from build123d import *

# Parameters (mm, degrees)
F0_R     = 6.5
F1_DEPTH = 60
F3_ANGLE = 90


# Not quite as in the source:
# - a feature names something its author has since deleted; it is built from what else it names


with BuildPart() as f1:
    # F0 (on Front) → F1 (new body)
    with BuildSketch(Plane.XZ):
        with BuildLine():
            Line((-11.7955299893, 45.4649311314), (-27.0527510662, 12.5336819647))
            ThreePointArc((-27.0527510662, 12.5336819647), (-29.8151727119, 0), (-27.0527510662, -12.5336819647))
            Line((-27.0527510662, -12.5336819647), (-11.7955299893, -45.4649311314))
            ThreePointArc((-11.7955299893, -45.4649311314), (0, -53), (11.7955299893, -45.4649311314))
            Line((11.7955299893, -45.4649311314), (27.0527510662, -12.5336819647))
            ThreePointArc((27.0527510662, -12.5336819647), (29.8151727119, 0), (27.0527510662, 12.5336819647))
            Line((27.0527510662, 12.5336819647), (11.7955299893, 45.4649311314))
            ThreePointArc((11.7955299893, 45.4649311314), (0, 53), (-11.7955299893, 45.4649311314))
        make_face()
        with Locations((0, -40)):
            Circle(F0_R, mode=Mode.SUBTRACT)
        with BuildLine():
            ThreePointArc((17.9448621018, -5.4354782815), (-18.75, 0), (17.9448621018, 5.4354782815))
            ThreePointArc((17.9448621018, 5.4354782815), (24.1748678936, 5.401139318), (27.28, 0))
            ThreePointArc((27.28, 0), (24.1748678936, -5.401139318), (17.9448621018, -5.4354782815))
        make_face(mode=Mode.SUBTRACT)
        with Locations((0, 40)):
            Circle(F0_R, mode=Mode.SUBTRACT)
        with BuildLine():
            ThreePointArc((17.9448621018, 5.4354782815), (18.5476233573, 2.7473929089), (18.75, 0))
            ThreePointArc((18.75, 0), (18.5476233573, -2.7473929089), (17.9448621018, -5.4354782815))
            ThreePointArc((17.9448621018, -5.4354782815), (24.1748678936, -5.401139318), (27.28, 0))
            ThreePointArc((27.28, 0), (24.1748678936, 5.401139318), (17.9448621018, 5.4354782815))
        make_face()
    extrude(amount=F1_DEPTH)


with BuildPart() as f2:
    # F0 (on Front) → F2 (revolve)
    with BuildSketch(Plane.XZ):
        with BuildLine():
            ThreePointArc((78.6849431597, 21.03), (68.9626292834, 15.8333148696), (70.0431715295, 26.8042470045))
            Line((70.0431715295, 26.8042470045), (65.4349431597, 24.8954563152))
            Line((65.4349431597, 24.8954563152), (65.4349431597, 0))
            Line((65.4349431597, 0), (79.4349431597, 0))
            Line((79.4349431597, 0), (79.4349431597, 24.8954563152))
            Line((79.4349431597, 24.8954563152), (74.8267146878, 26.8042470468))
            ThreePointArc((74.8267146878, 26.8042470468), (77.6316282594, 24.5023139222), (78.6849431597, 21.03))
        make_face()
        with BuildLine():
            ThreePointArc((74.8267146878, 26.8042470468), (72.4349431044, 27.28), (70.0431715295, 26.8042470045))
            ThreePointArc((70.0431715295, 26.8042470045), (68.9626292834, 15.8333148696), (78.6849431597, 21.03))
            ThreePointArc((78.6849431597, 21.03), (77.6316282594, 24.5023139222), (74.8267146878, 26.8042470468))
        make_face()
    revolve(axis=Axis((72.4349431597, 0, 0), (1, 0, 0)))


with BuildPart() as f2_1:
    # F3: moved
    add(f2.part.rotate(Axis((72.4349431597, 0, 17.3734594136), (0, 0, 1)), F3_ANGLE))


with BuildPart() as f2_2:
    # F4: moved
    add(f2_1.part.moved(Location((-72.7008, -12.31385, -0.07673))))


with BuildPart() as f1_1:
    add(f1.part)

    # F5: cut F2
    add(f2_2.part, mode=Mode.SUBTRACT)


solid = f1_1.part
The listing builds one solid part. Answer for the finished solid, in the listing's coordinates (mm). A direction names the side the tool comes from. Coordinates: 2 decimals unless noted, no trailing zeros. Loops run counter-clockwise (first coordinate to the right, second up) from the corner with the lowest first, then second, coordinate; pieces in that order, holes last. Notation, with made-up numbers: (-22, -29) -> (-14, -29) arc R24 ccw to (-14, -4) -> close; hole circle Ø10 at (-26.75, 41). An arc over 180 degrees is marked (long way). Write item = value, one per line. Start each with the question number.
1) A tool of negligible diameter and unlimited length cuts with its end or side. For faces 5 (the face through (16.4, -19.314, -9.4)), 6 (the face through (0, -30, -53)), from which of +Z, -Z, +X, -X, +Y, -Y can it reach the whole face along a straight path? Write none if from no direction.
2) A cutting plane is placed at C-C (z = -30). Give the vertices of the cut face in (x, y).
3) Given pin 1 Ø2 at (y, z) = (-32, 38) entering from -X; pin 2 Ø3 at (y, z) = (-21, 33.5) entering from -X; pin 3 Ø3 at (y, z) = (-8.5, 37) entering from -X, each flat-ended and moving along its own axis, determine where each tip first touches the part or whether it passes through.
4) Straight lines are drawn through the part: line 1 (Y direction, x = -0.5, z = 22); line 2 (X direction, y = -5.5, z = 13.5); line 3 (Z direction, x = -11, y = -44). For each, find the intervals that lie inside material, in ascending order. Write a range as from..to.
5) A cutting plane is placed at A-A (z = 36.5). Give the vertices of the cut face in (x, y), then the cut area to 3 significant figures.
6) The mould has two halves that part along X. Classify faces 1 (the face through (-20, -60, 1)), 2 (the face through (-19.53, -29.58, -28.77)), 3 (the face through (24.51, -19.09, -3.33)), 4 (the face through (-9, -5.314, 17)): released by +X, released by -X, zero draft, split by the parting line, or undercut.
7) A cutting plane is placed at B-B (x = 3.5). Count the separate pieces of the cut face and the enclosed holes in it, then the cut area to 3 significant figures.
Responses:
q1.face_5 = none
q1.face_6 = -Z, +Y, -Y
q2.outline = (-18.96, -60) -> (18.96, -60) -> (18.96, 0) -> (-18.96, 0) -> close
q3.pin_1 = -15.72
q3.pin_2 = -18.03
q3.pin_3 = -16.41
q4.line_1 = -60..-19.31, -5.31..0
q4.line_2 = -26.61..-21.23, 20.69..26.61
q4.line_3 = -46.93..-15.18, 15.18..46.93
q5.outline = (-15.95, -60) -> (-5.48, -60) -> (-5.48, 0) -> (-15.95, 0) -> close; (5.48, -60) -> (15.95, -60) -> (15.95, 0) -> (5.48, 0) -> close
q5.area = 1,260 mm²
q6.face_1 = zero draft
q6.face_2 = released by -X
q6.face_3 = undercut
q6.face_4 = undercut
q7.separate_pieces = 4
q7.enclosed_holes = 0
q7.area = 2,560 mm²
